```python
from build123d import *

# Parameters (mm, degrees)
ESBO_O1_R                = 1.5
ESBO_O1_R_2              = 3.5
ESBO_O1_R_3              = 0.9
ESBO_O1_W                = 22.6
ESBO_O1_H                = 12.3
ESBO_O1_W_2              = 3
ESBO_O1_H_2              = 8
ESBO_O1_W_3              = 8
ESBO_O1_H_3              = 3
RESSALTO_EXTRUS_O1_DEPTH = 3


with BuildPart() as part:
    # Esboço1 → Ressalto-extrusão1 (new body)
    with BuildSketch(Plane(origin=(0, 0, 0), x_dir=(1, 0, 0), z_dir=(0, 1, 0))):
        with BuildLine():
            Line((-4.674449837, 5.126823449), (2.15649844, 5.74992269))
            add(Edge.make_bspline(
                [(19.127700004, 3.859391667), (13.692888976, 5.757269931), (8.035822873, 6.387450044), (2.15649844, 5.74992269)],
                knots=[0.35388944, 0.35388944, 0.35388944, 0.35388944, 1, 1, 1, 1], degree=3))
            ThreePointArc((19.127700004, 3.859391667), (21.595587829, 3.06871935), (24.101127023, 2.406974398))
            add(Edge.make_bspline(
                [(24.101129521, -3.20712694), (35.966754752, -0.40007519), (24.101127023, 2.406974398)],
                knots=[5.194112275, 5.194112275, 5.194112275, 7.372258742, 7.372258742, 7.372258742], degree=2, weights=[1, 0.463306864, 1]))
            ThreePointArc((24.101129521, -3.20712694), (21.595589041, -3.868872862), (19.127700004, -4.659546287))
            add(Edge.make_bspline(
                [(19.127700004, -4.659546287), (13.692889505, -6.55742607), (8.035822337, -7.187603127), (2.15649844, -6.55007731)],
                knots=[0.35388944, 0.35388944, 0.35388944, 0.35388944, 1, 1, 1, 1], degree=3))
            Line((2.15649844, -6.55007731), (-4.674449837, -5.926978069))
            add(Edge.make_bspline(
                [(-23.759026807, -13.92609603), (-18.993134449, -8.145749128), (-12.424143506, -5.367564321), (-4.674449837, -5.926978069)],
                knots=[0.101821695, 0.101821695, 0.101821695, 0.101821695, 1, 1, 1, 1], degree=3))
            ThreePointArc((-23.759026807, -13.92609603), (-25.800414194, -15.798822034), (-28.277263571, -17.039621097))
            add(Edge.make_bspline(
                [(-28.277263571, -17.039621097), (-34.579205058, -19.166234), (-47.597806191, -22.747709276), (-59.650258973, -23.294853785), (-64.986052109, -22.387135922)],
                knots=[0.241589655, 0.241589655, 0.241589655, 0.241589655, 0.401358205, 0.561126756, 0.561126756, 0.561126756, 0.561126756], degree=3))
            ThreePointArc((-64.986052109, -22.387135922), (-69.209775007, -20.602207926), (-72.192804257, -17.119774932))
            ThreePointArc((-72.192804257, -17.119774932), (-76.257665323, -0.40007754), (-72.192804468, 16.319619904))
            ThreePointArc((-72.192804468, 16.319619904), (-69.209774999, 19.802053128), (-64.986051746, 21.586981094))
            add(Edge.make_bspline(
                [(-28.2772637, 16.239466453), (-34.57920511, 18.366079177), (-47.597806077, 21.947554059), (-59.650258689, 22.494698656), (-64.986051746, 21.586981094)],
                knots=[0.241589656, 0.241589656, 0.241589656, 0.241589656, 0.401358204, 0.561126752, 0.561126752, 0.561126752, 0.561126752], degree=3))
            ThreePointArc((-28.2772637, 16.239466453), (-25.80041422, 14.998667392), (-23.759026751, 13.125941342))
            add(Edge.make_bspline(
                [(-23.759026751, 13.125941342), (-18.993134399, 7.345594488), (-12.424143468, 4.567409699), (-4.674449837, 5.126823449)],
                knots=[0.101821698, 0.101821698, 0.101821698, 0.101821698, 1, 1, 1, 1], degree=3))
        make_face()
        with Locations((-59.742023738, -0.40007731)):
            Circle(ESBO_O1_R, mode=Mode.SUBTRACT)
        with Locations((-31.142023738, -0.40007731)):
            Circle(ESBO_O1_R, mode=Mode.SUBTRACT)
        with Locations((-45.242023738, 13.89992269)):
            Circle(ESBO_O1_R, mode=Mode.SUBTRACT)
        with Locations((-68.242023738, -14.70007731)):
            Circle(ESBO_O1_R, mode=Mode.SUBTRACT)
        with Locations((-59.742023738, 11.09992269)):
            Circle(ESBO_O1_R, mode=Mode.SUBTRACT)
        with Locations((-31.142023738, -11.40175485)):
            Circle(ESBO_O1_R, mode=Mode.SUBTRACT)
        with Locations((10.857976262, -0.40007731)):
            Circle(ESBO_O1_R_2, mode=Mode.SUBTRACT)
        with Locations((20.857976262, -0.40007731)):
            Circle(ESBO_O1_R_3, mode=Mode.SUBTRACT)
        with Locations((0.857976262, -0.40007731)):
            Circle(ESBO_O1_R_3, mode=Mode.SUBTRACT)
        with Locations((-14.142023738, -0.40007731)):
            Circle(ESBO_O1_R, mode=Mode.SUBTRACT)
        with Locations((-45.442023738, -0.40007731)):
            Rectangle(ESBO_O1_W, ESBO_O1_H, mode=Mode.SUBTRACT)
        with Locations((-45.242023738, -14.70007731)):
            Rectangle(ESBO_O1_W_2, ESBO_O1_H_2, mode=Mode.SUBTRACT)
        with Locations((-68.242023738, 13.89992269)):
            Rectangle(ESBO_O1_W_2, ESBO_O1_H_2, mode=Mode.SUBTRACT)
        with Locations((-31.142023738, 11.099922699)):
            Rectangle(ESBO_O1_W_3, ESBO_O1_H_3, mode=Mode.SUBTRACT)
        with Locations((-59.742023738, -11.90007731)):
            Rectangle(ESBO_O1_W_3, ESBO_O1_H_3, mode=Mode.SUBTRACT)
    extrude(amount=RESSALTO_EXTRUS_O1_DEPTH)


solid = part.part
```
Work out the finished part from the listing and answer in its coordinate system (mm). A direction names the side the tool comes from. Give positions to 0.01 mm unless a question says otherwise; leave off trailing zeros. One line per item, written item: value. Start each with the question number.
1. Consider line 1 (X direction, y = 0.35, z = 13.5); line 2 (Z direction, x = 11, y = 0.3); line 3 (Z direction, x = -62, y = 0.35). Determine where each line is inside the solid, lowest interval first.
2. Section A-A, the plane y = 1.7 is taken. Count the separate pieces of the cut face and the enclosed holes in it, then the cut area to 3 significant figures.
3. Each of these flat-tipped pins is pushed along its axis until it touches: pin 1 Ø1.5 at (x, y) = (-45.5, 1) entering from +Z; pin 2 Ø1.5 at (y, z) = (2, 9) entering from +X; pin 3 Ø4 at (x, z) = (10.86, 0.4) entering from -Y; pin 4 Ø0.9 at (x, y) = (-31, 1) entering from +Z. Where does it stop, or does it pass through?
4. Which of the six approach directions +Z, -Z, +X, -X, +Y, -Y give full straight-line access (tool end or side, diameter ignored) to faces 1 (the face through (-25.8, 1.5, 15.8)), 2 (the face through (-69.742, 1, -14))?
Filled sheet:
1. line 1: -73.82 to -69.14, -67.34 to -46.74, -43.74 to -23.4
1. line 2: -5.73 to -3.1, 3.9 to 6.53
1. line 3: -21.97 to 10.4, 13.4 to 22.77
2. separate pieces: 1
2. enclosed holes: 15
2. area: 2,200 mm²
3. pin 1: z = 21.8
3. pin 2: x = -16.83
3. pin 3: through
3. pin 4: z = 18.08
4. face 1: +Z, +X, +Y, -Y
4. face 2: +Y, -Y
